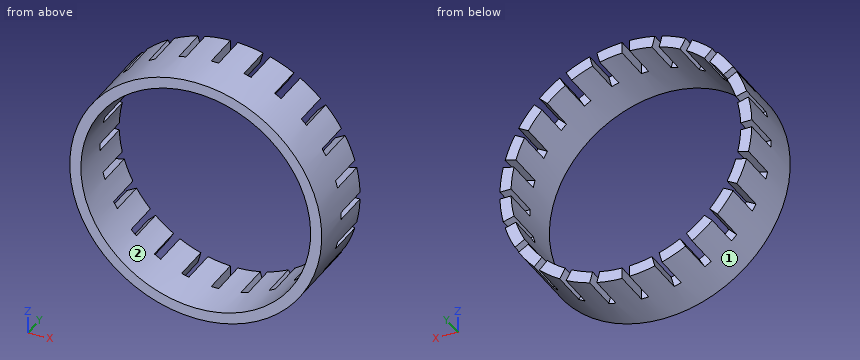
from build123d import *

# Parameters (mm, degrees)
SKETCH1_W          = 3
SKETCH1_H          = 20
SKETCH2_W          = 2
SKETCH2_H          = 38.722689076
CUT_EXTRUDE1_DEPTH = 40
CIRPATTERN1_COUNT  = 24


with BuildPart() as part:
    # Sketch1 → Revolve1 (revolve)
    with BuildSketch(Plane.XY, mode=Mode.PRIVATE) as revolve1_sk:
        with Locations((-32.5, 10)):
            Rectangle(SKETCH1_W, SKETCH1_H)
    revolve(revolve1_sk.sketch.rotate(Axis((0, -1.909188309, 0), (0, 1, 0)), 270), axis=Axis((0, -1.909188309, 0), (0, 1, 0)))

    # Sketch2 → Cut-Extrude1 (cut)
    with BuildSketch(Plane.XY):
        with Locations((0, 29.361344538)):
            Rectangle(SKETCH2_W, SKETCH2_H)
    cut_extrude1 = extrude(amount=-CUT_EXTRUDE1_DEPTH, mode=Mode.SUBTRACT)

    # CirPattern1: Cut-Extrude1 ×24 about axis
    cirpattern1_axis = Axis((0, 0, 0), (0, 1, 0))
    for i in range(1, CIRPATTERN1_COUNT):
        add(cut_extrude1.rotate(cirpattern1_axis, i * 360 / CIRPATTERN1_COUNT), mode=Mode.SUBTRACT)


solid = part.part
Design review of the part built by this model. Coordinates are the model's own, in mm. Face numbers are marked on the shaded views. Give positions to 0.01 mm unless a question says otherwise; leave off trailing zeros. Order: outer loops, then holes, each group sorted by start corner. A loop starts at its lowest first (then second) coordinate and runs counter-clockwise, first axis right, second up.
1. Add section B-B, the plane x = 0. State the section outline as (y, z) points.
Solution:
outline: (0, -34) - (10, -34) - (10, -31) - (0, -31) - close; (0, 31) - (10, 31) - (10, 34) - (0, 34) - close
2. To check wall thickness, follow L1, parallel to X at y = 6.25, z = 0; L2, parallel to X at y = 7.25, z = -21; L3, parallel to Z at x = -19.5, y = 15.5. State the ranges of each line that lie inside material, in increasing order.
Solution:
L1: x = -34 to -31, 31 to 34
L2: x = -26.74 to -22.8, 22.8 to 26.74
L3: z = -27.85 to -24.1, 24.1 to 27.85
3. For pin 1 Ø3.5 at (x, y) = (-33, 13.5) entering from +Z; pin 2 Ø1.6 at (x, z) = (-27.5, -16) entering from +Y; pin 3 Ø10 at (y, z) = (11.5, 20.5) entering from +X, all flat-tipped, find the tip position at first contact; note any pin that passes through.
Solution:
pin 1: stops at z = 13.4
pin 2: stops at y = 10
pin 3: stops at x = 30.26
4. Add section A-A, the plane z = 0. State the section outline as (x, y) points.
Solution:
outline: (-34, 0) - (-31, 0) - (-31, 10) - (-34, 10) - close; (31, 0) - (34, 0) - (34, 10) - (31, 10) - close
5. Add section D-D, the plane y = 7.25. State the section outline as (x, z) points.
Solution:
outline: circle Ø68 at (0, 0); hole circle Ø62 at (0, 0)
6. Mouldability with a two-part tool opening along X and no side actions: class the marked faces 1 and 2 as +X half, -X half, draft (parallel to the pull), parting line (faces both ways), or undercut.
Solution:
face 1: parting line
face 2: undercut
7. Add section C-C, the plane y = 13.5. State how many separate pieces and enclosed holes the cut face has, then the cut area to 3 significant figures.
Solution:
separate pieces: 24
enclosed holes: 0
area: 469 mm2
